from build123d import *

# Parameters (mm, degrees)
BOSS_EXTRUDE1_DEPTH     = 13
SKETCH6_W               = 6
SKETCH6_H               = 5
BOSS_EXTRUDE4_DEPTH     = 5.6
SKETCH16_W              = 6
SKETCH16_H              = 8
BOSS_EXTRUDE5_DEPTH     = 0.1
CUT_EXTRUDE6_DEPTH      = 4
CUT_EXTRUDE6_DEPTH_BACK = 3.6
SKETCH15_R              = 1.3
CUT_EXTRUDE7_DEPTH      = 8.7202
CUT_EXTRUDE8_START      = -0.2202
SKETCH19_W              = 6
SKETCH19_H              = 8
SKETCH19_R              = 1.3
CUT_EXTRUDE8_DEPTH      = 0.2202
SKETCH12_R              = 1.2
CUT_EXTRUDE5_DEPTH      = 6
SKETCH21_R              = 1.2
BOSS_EXTRUDE6_DEPTH     = 2.5
SKETCH24_W              = 6
SKETCH24_H              = 5.5
CUT_EXTRUDE10_DEPTH     = 8.5
BOSS_EXTRUDE8_DEPTH     = 7.2
FILLET4_R               = 1.5
SKETCH26_R              = 1.3
CUT_EXTRUDE11_DEPTH     = 10
CHAMFER1_SIZE           = 0.2
BOSS_EXTRUDE9_DEPTH     = 5
SKETCH31_R              = 1.3
CUT_EXTRUDE12_DEPTH     = 8
CROQUIS1_W              = 20.968017067
CROQUIS1_H              = 19.092350392
CORTAR_EXTRUIR1_DEPTH   = 0.5
CORTAR_EXTRUIR2_DEPTH   = 2


with BuildPart() as part:
    # Sketch1 → Boss-Extrude1 (new body)
    with BuildSketch(Plane.XY):
        Polygon((3, 3.05), (3, -2.253801214), (2.388188946, -2.95), (-2.388188946, -2.95), (-3, -2.253801214), (-3, 3.05), align=None)
    extrude(amount=BOSS_EXTRUDE1_DEPTH)

    # Sketch6 → Boss-Extrude4 (add)
    with BuildSketch(Plane(origin=(0, 3.05, 0), x_dir=(1, 0, 0), z_dir=(0, 1, 0))):
        with Locations((0, -2.5)):
            Rectangle(SKETCH6_W, SKETCH6_H)
    extrude(amount=BOSS_EXTRUDE4_DEPTH)

    # Sketch16 → Boss-Extrude5 (add)
    with BuildSketch(Plane(origin=(0, 3.05, 0), x_dir=(1, 0, 0), z_dir=(0, 1, 0))):
        with Locations((0, -9)):
            Rectangle(SKETCH16_W, SKETCH16_H)
    extrude(amount=BOSS_EXTRUDE5_DEPTH)

    # Sketch18 → Cut-Extrude6 (cut, two sides: drawn at the far end of the back side and taken through both)
    with BuildSketch(Plane(origin=(0, 0, 0), x_dir=(0, 0, -1), z_dir=(1, 0, 0)).offset(-CUT_EXTRUDE6_DEPTH_BACK)):
        with BuildLine():
            Line((-8.8572, -0.0702), (-12.8572, -0.0702))
            Line((-12.8572, -0.0702), (-13, -0.0702))
            Line((-13, -0.0702), (-13, -0.7))
            Line((-13, -0.7), (-12.8572, -0.7))
            Line((-12.8572, -0.7), (-12.7144, -0.7))
            add(Edge.make_bspline(
                [(-12.7144, -0.7), (-12.5198, -0.7), (-12.43, -0.9509)],
                knots=[0.103448276, 0.103448276, 0.103448276, 0.137931034, 0.137931034, 0.137931034], degree=2))
            add(Edge.make_bspline(
                [(-12.43, -0.9509), (-12.3594, -1.2388), (-12.13, -1.45), (-11.8572, -1.45)],
                knots=[0.137931034, 0.137931034, 0.137931034, 0.137931034, 0.172413793, 0.172413793, 0.172413793, 0.172413793], degree=3))
            add(Edge.make_bspline(
                [(-11.8572, -1.45), (-11.5844, -1.45), (-11.355, -1.2388), (-11.2844, -0.9509)],
                knots=[0.172413793, 0.172413793, 0.172413793, 0.172413793, 0.206896552, 0.206896552, 0.206896552, 0.206896552], degree=3))
            add(Edge.make_bspline(
                [(-11.2844, -0.9509), (-11.1946, -0.7), (-11, -0.7)],
                knots=[0.206896552, 0.206896552, 0.206896552, 0.24137931, 0.24137931, 0.24137931], degree=2))
            Line((-11, -0.7), (-10.8572, -0.7))
            Line((-10.8572, -0.7), (-10.7144, -0.7))
            add(Edge.make_bspline(
                [(-10.7144, -0.7), (-10.5198, -0.7), (-10.43, -0.9509)],
                knots=[0.310344828, 0.310344828, 0.310344828, 0.344827586, 0.344827586, 0.344827586], degree=2))
            add(Edge.make_bspline(
                [(-10.43, -0.9509), (-10.3594, -1.2388), (-10.13, -1.45), (-9.8572, -1.45)],
                knots=[0.344827586, 0.344827586, 0.344827586, 0.344827586, 0.379310345, 0.379310345, 0.379310345, 0.379310345], degree=3))
            add(Edge.make_bspline(
                [(-9.8572, -1.45), (-9.5844, -1.45), (-9.355, -1.2388), (-9.2844, -0.9509)],
                knots=[0.379310345, 0.379310345, 0.379310345, 0.379310345, 0.413793103, 0.413793103, 0.413793103, 0.413793103], degree=3))
            add(Edge.make_bspline(
                [(-9.2844, -0.9509), (-9.1946, -0.7), (-9, -0.7)],
                knots=[0.413793103, 0.413793103, 0.413793103, 0.448275862, 0.448275862, 0.448275862], degree=2))
            Line((-9, -0.7), (-8.8572, -0.7))
            Line((-8.8572, -0.7), (-8.7144, -0.7))
            add(Edge.make_bspline(
                [(-8.7144, -0.7), (-8.5198, -0.7), (-8.43, -0.9509)],
                knots=[0.517241379, 0.517241379, 0.517241379, 0.551724138, 0.551724138, 0.551724138], degree=2))
            add(Edge.make_bspline(
                [(-8.43, -0.9509), (-8.3594, -1.2388), (-8.13, -1.45), (-7.8572, -1.45)],
                knots=[0.551724138, 0.551724138, 0.551724138, 0.551724138, 0.586206897, 0.586206897, 0.586206897, 0.586206897], degree=3))
            add(Edge.make_bspline(
                [(-7.8572, -1.45), (-7.5844, -1.45), (-7.355, -1.2388), (-7.2844, -0.9509)],
                knots=[0.586206897, 0.586206897, 0.586206897, 0.586206897, 0.620689655, 0.620689655, 0.620689655, 0.620689655], degree=3))
            add(Edge.make_bspline(
                [(-7.2844, -0.9509), (-7.1946, -0.7), (-7, -0.7)],
                knots=[0.620689655, 0.620689655, 0.620689655, 0.655172414, 0.655172414, 0.655172414], degree=2))
            Line((-7, -0.7), (-6.8572, -0.7))
            Line((-6.8572, -0.7), (-6.7144, -0.7))
            add(Edge.make_bspline(
                [(-6.7144, -0.7), (-6.5198, -0.7), (-6.43, -0.9509)],
                knots=[0.724137931, 0.724137931, 0.724137931, 0.75862069, 0.75862069, 0.75862069], degree=2))
            add(Edge.make_bspline(
                [(-6.43, -0.9509), (-6.3594, -1.2388), (-6.13, -1.45), (-5.8572, -1.45)],
                knots=[0.75862069, 0.75862069, 0.75862069, 0.75862069, 0.793103448, 0.793103448, 0.793103448, 0.793103448], degree=3))
            add(Edge.make_bspline(
                [(-5.8572, -1.45), (-5.5844, -1.45), (-5.355, -1.2388), (-5.2844, -0.9509)],
                knots=[0.793103448, 0.793103448, 0.793103448, 0.793103448, 0.827586207, 0.827586207, 0.827586207, 0.827586207], degree=3))
            add(Edge.make_bspline(
                [(-5.2844, -0.9509), (-5.1946, -0.7), (-5, -0.7)],
                knots=[0.827586207, 0.827586207, 0.827586207, 0.862068966, 0.862068966, 0.862068966], degree=2))
            Line((-5, -0.7), (-5, -0.0702))
            Line((-5, -0.0702), (-8.8572, -0.0702))
        make_face()
    extrude(amount=CUT_EXTRUDE6_DEPTH + CUT_EXTRUDE6_DEPTH_BACK, mode=Mode.SUBTRACT)

    # Sketch15 → Cut-Extrude7 (cut)
    with BuildSketch(Plane(origin=(0, 8.65, 0), x_dir=(1, 0, 0), z_dir=(0, 1, 0))):
        with Locations(Location((0, -10.8572, 0), (0, 0, 180))):
            Circle(SKETCH15_R)
        with Locations(Location((0, -6.8572, 0), (0, 0, 180))):
            Circle(SKETCH15_R)
    extrude(amount=-CUT_EXTRUDE7_DEPTH, mode=Mode.SUBTRACT)

    # Sketch19 → Cut-Extrude8 (cut)
    with BuildSketch(Plane.XZ.offset(0.0702).offset(CUT_EXTRUDE8_START)):
        with Locations((0, 9)):
            Rectangle(SKETCH19_W, SKETCH19_H)
        with Locations(Location((0, 10.8572, 0), (0, 0, 180))):
            Circle(SKETCH19_R, mode=Mode.SUBTRACT)
        with Locations(Location((0, 6.8572, 0), (0, 0, 180))):
            Circle(SKETCH19_R, mode=Mode.SUBTRACT)
    extrude(amount=CUT_EXTRUDE8_DEPTH, mode=Mode.SUBTRACT)

    # Sketch12 → Cut-Extrude5 (cut)
    with BuildSketch(Plane.XY.offset(5)):
        with Locations((0, 5.85)):
            Circle(SKETCH12_R)
    extrude(amount=-CUT_EXTRUDE5_DEPTH, mode=Mode.SUBTRACT)

    # Sketch21 → Boss-Extrude6 (add)
    with BuildSketch(Plane(origin=(0, 0, 0), x_dir=(-1, 0, 0), z_dir=(0, 0, -1))):
        Polygon((-2.388188946, -2.95), (2.388188946, -2.95), (3, -2.253801214), (3, 8.65), (-3, 8.65), (-3, -2.253801214), align=None)
        with Locations(Location((0, 5.85, 0), (0, 0, 180))):
            Circle(SKETCH21_R, mode=Mode.SUBTRACT)
    extrude(amount=BOSS_EXTRUDE6_DEPTH)

    # Sketch24 → Cut-Extrude10 (cut)
    with BuildSketch(Plane.XY.offset(5)):
        with Locations((0, 5.9)):
            Rectangle(SKETCH24_W, SKETCH24_H)
    extrude(amount=-CUT_EXTRUDE10_DEPTH, mode=Mode.SUBTRACT)

    # Sketch25 → Boss-Extrude8 (add)
    with BuildSketch(Plane(origin=(0, 3.15, 0), x_dir=(1, 0, 0), z_dir=(0, 1, 0))):
        Polygon((-10, -4.5), (0, -4.5), (3.5, -4.5), (3.5, 2.5), (-10, 2.5), align=None)
    extrude(amount=BOSS_EXTRUDE8_DEPTH)

    # Fillet4
    fillet4_edges = [part.edges().sort_by_distance(p)[0] for p in [
        (-10, 3.15, 1),
    ]]
    fillet(fillet4_edges, radius=FILLET4_R)

    # Sketch26 → Cut-Extrude11 (cut)
    with BuildSketch(Plane.XY.offset(4.5)):
        with Locations((0, 5.9)):
            Circle(SKETCH26_R)
    extrude(amount=-CUT_EXTRUDE11_DEPTH, mode=Mode.SUBTRACT)

    # Chamfer1
    chamfer1_edges = [part.edges().sort_by_distance(p)[0] for p in [
        (-2.694094473, -2.601900607, 13),
        (0, -2.95, 13),
        (2.694094473, -2.601900607, 13),
        (3, 1.65, 13),
        (3, -1.476900607, 13),
        (-3, -1.476900607, 13),
        (-3, 1.65, 13),
    ]]
    chamfer(chamfer1_edges, length=CHAMFER1_SIZE)

    # Sketch29 → Boss-Extrude9 (add)
    with BuildSketch(Plane(origin=(0, 0, -2.5), x_dir=(-1, 0, 0), z_dir=(0, 0, -1))):
        with BuildLine():
            Line((3.53, 3.15), (3.53, 10.35))
            Line((3.53, 10.35), (10, 10.35))
            Line((10, 10.35), (10, 4.65))
            ThreePointArc((10, 4.65), (9.560660172, 3.589339828), (8.5, 3.15))
            Line((8.5, 3.15), (3.53, 3.15))
        make_face()
    extrude(amount=BOSS_EXTRUDE9_DEPTH)

    # Sketch31 → Cut-Extrude12 (cut)
    with BuildSketch(Plane(origin=(0, 10.35, 0), x_dir=(1, 0, 0), z_dir=(0, 1, 0))):
        with Locations(Location((-6.765, 4.5, 0), (0, 0, 180))):
            Circle(SKETCH31_R)
        with Locations(Location((-6.765, -1.1, 0), (0, 0, 180))):
            Circle(SKETCH31_R)
    extrude(amount=-CUT_EXTRUDE12_DEPTH, mode=Mode.SUBTRACT)

    # Croquis1 → Cortar-Extruir1 (cut)
    with BuildSketch(Plane(origin=(3.5, 0, 0), x_dir=(0, 0, -1), z_dir=(1, 0, 0))):
        with Locations((-1.115538408, 6.705636454)):
            Rectangle(CROQUIS1_W, CROQUIS1_H)
    extrude(amount=-CORTAR_EXTRUIR1_DEPTH, mode=Mode.SUBTRACT)

    # Croquis2 → Cortar-Extruir2 (cut)
    with BuildSketch(Plane.XY.offset(4.5)):
        Polygon((1.58771324, 8.65), (-1.58771324, 8.65), (-3.175426481, 5.9), (-1.58771324, 3.15), (1.58771324, 3.15), (3.175426481, 5.9), align=None)
    extrude(amount=-CORTAR_EXTRUIR2_DEPTH, mode=Mode.SUBTRACT)


solid = part.part
Can you work these out from the model? Positions are in its coordinate system, mm. A direction names the side the tool comes from. Give positions to 0.01 mm unless a question says otherwise; leave off trailing zeros. Loops run counter-clockwise (first coordinate to the right, second up) from the corner with the lowest first, then second, coordinate; pieces in that order, holes last. Notation, with made-up numbers: (5, -6.75) - (19, -6.75) arc R9 cw to (19, 0.25) - close; hole circle Ø10 at (3.5, 82). An arc over 180 degrees is marked (long way). Return JSON: item names as keys, results as strings.
1. If I drill on line 1 (Z direction, x = 0, y = 1.7); line 2 (Y direction, x = 0, z = 0.15); line 3 (X direction, y = 5.5, z = 1.5), over which ranges is the centre line in solid material (lowest first)?
Output values:
{"line 1": "z = -2.5 to 5.56, 8.16 to 9.56, 12.16 to 13", "line 2": "y = -2.95 to 4.6, 7.2 to 10.35", "line 3": "x = -10 to -8, -5.53 to -1.24, 1.24 to 3"}
2. I want a section at C-C on y = 1.5. Please give me the cut outline in (x, z).
Output values:
{"outline": "(-3, -2.5) - (3, -2.5) - (3, 12.8) - (2.8, 13) - (-2.8, 13) - (-3, 12.8) - close; hole circle Ø2.6 at (0, 6.86); hole circle Ø2.6 at (0, 10.86)"}
3. I'm going to push flat-ended pins straight in: pin 1 Ø4.5 at (y, z) = (0.5, 8.5) entering from -X; pin 2 Ø5 at (x, z) = (-0.5, 7.5) entering from +Y; pin 3 Ø1 at (x, y) = (-6, 7) entering from +Z. Where does each tip first touch, or does it pass through?
Output values:
{"pin 1": "stops at x = -3", "pin 2": "stops at y = 3.15", "pin 3": "stops at z = 4.5"}
4. I want a section at A-A on z = 1.1. Please give me the cut outline in (x, y) (3 decimals).
Output values:
{"outline": "(-10, 4.65) arc R1.5 ccw to (-8.5, 3.15) - (-8.065, 3.15) - (-8.065, 10.35) - (-10, 10.35) - close; (-5.465, 3.15) - (-3, 3.15) - (-3, -2.254) - (-2.388, -2.95) - (2.388, -2.95) - (3, -2.254) - (3, 10.35) - (-5.465, 10.35) - close; hole circle Ø2.6 at (0, 5.9)"}
5. I want a section at B-B on x = -6.25. Please give me the cut outline in (y, z), and give its area (3 significant figures).
Output values:
{"outline": "(3.15, -7.5) - (10.35, -7.5) - (10.35, -5.69) - (3.15, -5.69) - close; (3.15, -3.31) - (10.35, -3.31) - (10.35, -0.09) - (3.15, -0.09) - close; (3.15, 2.29) - (10.35, 2.29) - (10.35, 4.5) - (3.15, 4.5) - close", "area": "52.0 mm²"}
6. We'd pull the mould along Z, two halves only. Please class faces 1 (the face through (0.282, 1.671, 5.588)), 2 (the face through (-6, 3.15, -1)), 3 (the face through (1, 7, 2.5)): +Z half, -Z half, draft (parallel to the pull), parting line (faces both ways), or undercut.
Output values:
{"face 1": "undercut", "face 2": "draft", "face 3": "+Z half"}
7. I want a section at D-D on z = -5.25. Please give me the cut outline in (x, y).
Output values:
{"outline": "(-10, 4.65) arc R1.5 ccw to (-8.5, 3.15) - (-7.83, 3.15) - (-7.83, 10.35) - (-10, 10.35) - close; (-5.7, 3.15) - (-3.53, 3.15) - (-3.53, 10.35) - (-5.7, 10.35) - close"}
8. For faces 4 (the face through (2.6, 3.8, 4.5)), 5 (the face through (0, 0.15, 9)), 6 (the face through (0, 3.15, 9)), 7 (the face through (-8, 6.8, 1.5)), which set-ups out of +Z, -Z, +X, -X, +Y, -Y let a thin tool reach every point of the face, with its end or its side?
Output values:
{"face 4": "+Z, +X, -X, +Y", "face 5": "+Z, +X, -X", "face 6": "+Z", "face 7": "+Y, -Y"}
